Autodesk Inventor part; units mm, degrees
ref_plane "YZ Plane" through (0, 0, 0) normal (1, 0, 0) x (0, 1, 0)
ref_plane "XZ Plane" through (0, 0, 0) normal (0, 1, 0) x (-1, 0, 0)
ref_plane "XY Plane" through (0, 0, 0) normal (0, 0, 1) x (1, 0, 0)
sketch "スケッチ1" plane through (0, 0, 0) normal (0, 0, 1) x (1, 0, 0)
  line L0 (-100, 100) -> (100, 100)
  line L1 (100, 100) -> (100, -100)
  line L2 (100, -100) -> (-100, -100)
  line L3 (-100, -100) -> (-100, 100)
  line L4 (-100, 100) -> (100, -100) construction
  line L5 (100, 100) -> (-100, -100) construction
  circle A0 centre (0, 0) radius 92.5 construction
  circle A1 centre (-65.4074, 65.4074) radius 4
  circle A2 centre (65.4074, 65.4074) radius 4
  circle A3 centre (65.4074, -65.4074) radius 4
  circle A4 centre (-65.4074, -65.4074) radius 4
  dimension "d0" = 200
  dimension "d1" = 200
  dimension "d2" = 185
  dimension "d3" = 8
  dimension "d4" = 8
  dimension "d5" = 8
  dimension "d6" = 8
extrude "押し出し1" add sketch "スケッチ1" along normal blind 3
sketch "スケッチ2" plane through (0, 0, 0) normal (0, 0, -1) x (-1, 0, 0)
  circle A0 centre (0, 0) radius 72.5
  dimension "d9" = 145
extrude "押し出し2" cut sketch "スケッチ2" against normal blind 10
sketch "スケッチ3" plane through (0, 0, 3) normal (0, 0, 1) x (1, 0, 0)
  circle A0 centre (-65.4074, -65.4074) radius 4
  circle A1 centre (65.4074, -65.4074) radius 4
  point P0 (0, 0)
sketch "スケッチ4" plane through (-100, -100, 0) normal (0, -1, 0) x (1, 0, 0)
  line L0 (0, 0) -> (0, 3)
  line L1 (200, 0) -> (200, 3)
  line L2 (0, 3) -> (200, 3)
  line L3 (200, 3) -> (200, 0)
  line L4 (200, 0) -> (0, 0)
  line L5 (0, 0) -> (0, 3)
  point P0 (100, 0)
extrude "押し出し3" add sketch "スケッチ4" along normal blind 100
sketch "スケッチ7" plane through (0, 0, 0) normal (0, 0, -1) x (-1, 0, 0)
  circle A0 centre (30, -128) radius 3
  circle A1 centre (-30, -128) radius 3
  circle A2 centre (30, -102) radius 3
  circle A3 centre (-30, -102) radius 3
  point P0 (0, -115)
  dimension "d40" = 6
  dimension "d41" = 6
  dimension "d42" = 6
  dimension "d43" = 6
sketch "スケッチ8" plane through (-100, 100, 0) normal (0, 1, 0) x (1, 0, 0)
  line L0 (0, 0) -> (200, 0)
  line L1 (200, 0) -> (200, -3)
  line L2 (0, 0) -> (200, 0)
  line L3 (200, 0) -> (200, -3)
  line L4 (200, -3) -> (0, -3)
  line L5 (0, -3) -> (0, 0)
  point P0 (100, 0)
extrude "押し出し7" add sketch "スケッチ8" along normal blind 100
sketch "スケッチ9" plane through (0, 0, 0) normal (0, 0, -1) x (-1, 0, 0)
  circle A0 centre (0, -120) radius 30
  circle A1 centre (0, 0) radius 102.5
  circle A2 centre (0, -150) radius 1.65
  circle A3 centre (-45, -150) radius 1.65
  circle A4 centre (-90, -150) radius 1.65
  circle A5 centre (45, -150) radius 1.65
  circle A6 centre (90, -150) radius 1.65
  circle A7 centre (-90, 150) radius 1.65
  circle A8 centre (-45, 150) radius 1.65
  circle A9 centre (0, 150) radius 1.65
  circle A10 centre (45, 150) radius 1.65
  circle A11 centre (90, 150) radius 1.65
  dimension "d44" = 60
  dimension "d47" = 205
  dimension "d60" = 3.3
  dimension "d61" = 3.3
  dimension "d62" = 3.3
  dimension "d63" = 3.3
  dimension "d64" = 3.3
  dimension "d65" = 3.3
  dimension "d66" = 3.3
  dimension "d67" = 3.3
  dimension "d68" = 3.3
  dimension "d69" = 3.3
extrude "押し出し8" cut sketch "スケッチ7" against normal blind 10
sketch "スケッチ10" plane through (0, 0, 0) normal (0, 0, -1) x (-1, 0, 0)
  point P0 (0, 0)
sketch "スケッチ11" plane through (0, 0, 0) normal (0, 0, -1) x (-1, 0, 0)
  point P0 (0, 0)
extrude "押し出し10" cut sketch "スケッチ9" against normal blind 10 contours A2 A0 | A0 A2 | A3 | A4 | A5 | A6 | A7 | A8 | A9 | A10 | A11
sketch "スケッチ12" plane through (0, 0, 0) normal (0, 0, -1) x (-1, 0, 0)
  circle A0 centre (0, -150) radius 1.65
  circle A1 centre (0, -150) radius 7.5
  point P0 (0, 0)
  dimension "d72" = 15
sketch "スケッチ13" plane through (0, 0, 0) normal (0, 0, -1) x (-1, 0, 0)
  circle A0 centre (-90, -90) radius 1.65
  circle A1 centre (90, -90) radius 1.65
  circle A2 centre (-90, 90) radius 1.65
  circle A3 centre (90, 90) radius 1.65
  circle A4 centre (-90, -120) radius 1.65
  circle A5 centre (90, -120) radius 1.65
  circle A6 centre (-90, 120) radius 1.65
  circle A7 centre (90, 120) radius 1.65
  point P0 (0, 0)
  dimension "d81" = 3.3
  dimension "d82" = 3.3
  dimension "d83" = 3.3
  dimension "d84" = 3.3
  dimension "d85" = 3.3
  dimension "d86" = 3.3
  dimension "d87" = 3.3
  dimension "d88" = 3.3
sketch "スケッチ14" plane through (0, 0, 0) normal (0, 0, -1) x (-1, 0, 0)
  circle A0 centre (0, 0) radius 92.5
  circle A1 centre (0, -92.5) radius 3
  circle A2 centre (-92.5, 0) radius 3
  circle A3 centre (0, 92.5) radius 3
  circle A4 centre (92.5, 0) radius 3
  dimension "d74" = 185
  dimension "d75" = 6
  dimension "d76" = 6
  dimension "d77" = 6
  dimension "d78" = 6
extrude "押し出し11" cut sketch "スケッチ14" against normal blind 10 contours A0 A4 | A0 A4 | A3 A0 | A0 A3 | A1 A0 | A0 A1 | A2 A0 | A0 A2
extrude "押し出し12" cut sketch "スケッチ13" against normal blind 10
properties part number "ベアリング板" material "アルミニウム 6061"
Design review of the part built by this model. Coordinates are the model's own, in mm. Give positions to 0.01 mm unless a question says otherwise; leave off trailing zeros. Order: outer loops, then holes, each group sorted by start corner. A loop starts at its lowest first (then second) coordinate and runs counter-clockwise, first axis right, second up. Notation, with made-up numbers: (-2, 10.25) - (53, 10.25) arc R27 ccw to (53, 45.25) - close; hole circle Ø3 at (3, 48). An arc over 180 degrees is marked (long way). Use a Markdown table: item, result. Add a question column.
(1) Add section B-B on x = -13.5. Give the boundary of the cut face in (y, z).
(2) Mouldability with a two-part tool opening along X and no side actions: class faces 1 (the face through (69.223, 64.206, 1.479)), 2 (the face through (68, 42, 3)) as +X half, -X half, draft (parallel to the pull), parting line (faces both ways), or undercut.
(3) Wall thickness on probe 1 along X at (y, z) = (-65, 1); probe 2 along X at (y, z) = (92.5, 1.8); probe 3 along Y at (x, z) = (29, 0.7): over which ranges is each line inside the solid? List them lowest first. Write a range as [from, to].
(4) Add section C-C on z = 1. Give the number of separate pieces and of enclosed holes in the cut face, then the cut area to 3 significant figures.
(5) Add section A-A on y = 48.5. Give the boundary of the cut face in (x, z), then the cut area to 3 significant figures.
(6) Clearance check with flat-ended pins moving along their axes: P1, Ø4.5, axis at x = 45, y = 150, coming from the +Z side; P2, Ø3, axis at x = 90, y = 150, coming from the -Z side. State where each tip first meets the part, or that it passes through.
Report:
| question | item | result |
|---|---|---|
| 1 | outline | (-200, 0) - (-71.23, 0) - (-71.23, 3) - (-200, 3) - close; (71.23, 0) - (200, 0) - (200, 3) - (71.23, 3) - close |
| 2 | face 1 | undercut |
| 2 | face 2 | draft |
| 3 | probe 1 | x = [-100, -69.39], [-61.43, -32.11], [32.11, 61.43], [69.39, 100] |
| 3 | probe 2 | x = [-100, -3], [3, 100] |
| 3 | probe 3 | y = [-200, -130.83], [-125.17, -104.83], [-99.17, -66.45], [66.45, 200] |
| 4 | separate pieces | 1 |
| 4 | enclosed holes | 31 |
| 4 | area | 62,900 mm² |
| 5 | outline | (-100, 0) - (-53.89, 0) - (-53.89, 3) - (-100, 3) - close; (53.89, 0) - (100, 0) - (100, 3) - (53.89, 3) - close |
| 5 | area | 277 mm² |
| 6 | P1 | stops at z = 3 |
| 6 | P2 | passes through |
